Part model, mm, in its own coordinate system. A direction names the side the tool comes from. Round coordinates to 2 decimals unless told otherwise and drop trailing zeros. Order: outer loops, then holes, each group sorted by start corner. A loop starts at its lowest first (then second) coordinate and runs counter-clockwise, first axis right, second up. Notation, with made-up numbers: (-8, 86) -> (11, 86) arc R23 ccw to (11, 107) -> close; hole circle Ø8 at (58, 33). An arc over 180 degrees is marked (long way). Answer as a JSON object with one key per item and string values. Group by question number.
```python
from build123d import *

# Parameters (mm, degrees)
F0_R     = 30
F1_DEPTH = 2
F2_W     = 3
F2_H     = 8


# Not quite as in the source:
# - the program builds the solid bodies; features that only make, move or delete a surface that nothing else refers to are left out


with BuildPart() as f1:
    # F0 (on Top) → F1 (new body)
    with BuildSketch(Plane.XY):
        Circle(F0_R)
    extrude(amount=F1_DEPTH)

    # F2 (on Front) → F3 (revolve)
    with BuildSketch(Plane.XZ):
        with Locations((24.5, 4)):
            Rectangle(F2_W, F2_H)
    revolve(axis=Axis((0, 0, 15.4871546511), (0, 0, 1)))


solid = f1.part
```
Q1. Which spindle directions (+Z, -Z, +X, -X, +Y, -Y) get a long thin tool onto all of the face, cutting with end or side? Do faces 1 (the cylindrical face through (-29.97, 1.32, 0.99)), 2 (the cylindrical face through (-2.994, 22.804, 5.042)). Say none if no direction does.
Q2. Band-saw the part on A-A (y = 0). List the corners of the cut face in (x, z).
Q3. Drop flat-ended pins along their axis: pin 1 Ø2 at (x, z) = (13, 4.5) entering from -Y; pin 2 Ø3 at (x, z) = (7.5, 1) entering from -Y; pin 3 Ø2 at (x, z) = (-2.5, 4) entering from +Y. Give the stop position or say it passes through.
Q4. Band-saw the part on C-C (z = 7). List the corners of the cut face in (x, y), plus the area to 3 significant figures.
Q5. Wall check: line 1 (Y direction, x = 0, z = 5.85); line 2 (Z direction, x = 11, y = 5); line 3 (X direction, y = 16.5, z = 4.25). Give the ranges that are in metal, low to high. Write a range as [from, to].
Q6. Two-plate mould, pull along Y, no slides. Class faces 3 (the cylindrical face through (-20.633, -15.821, 5.042)), 4 (the flat face through (0, 0, 2)), 5 (the flat face through (0, 0, 0)): +Y half, -Y half, draft (parallel to the pull), parting line (faces both ways), or undercut.
Completed:
{
 "1": {"face 1": "+Z, -Z", "face 2": "+Z"},
 "2": {"outline": "(-30, 0) -> (30, 0) -> (30, 2) -> (26, 2) -> (26, 8) -> (23, 8) -> (23, 2) -> (-23, 2) -> (-23, 8) -> (-26, 8) -> (-26, 2) -> (-30, 2) -> close"},
 "3": {"pin 1": "y = -23.07", "pin 2": "y = -29.39", "pin 3": "y = 25.96"},
 "4": {"outline": "circle Ø52 at (0, 0); hole circle Ø46 at (0, 0)", "area": "462 mm2"},
 "5": {"line 1": "[-26, -23], [23, 26]", "line 2": "[0, 2]", "line 3": "[-20.09, -16.02], [16.02, 20.09]"},
 "6": {"face 3": "parting line", "face 4": "undercut", "face 5": "draft"}
}
